The drawing under review shows one solid part. Ordinate dimensions are in mm from its lowest x, y, z. Coordinates: 2 decimals unless noted, no trailing zeros. Order: outer loops, then holes, each group sorted by start corner. A loop starts at its lowest first (then second) coordinate and runs counter-clockwise, first axis right, second up.
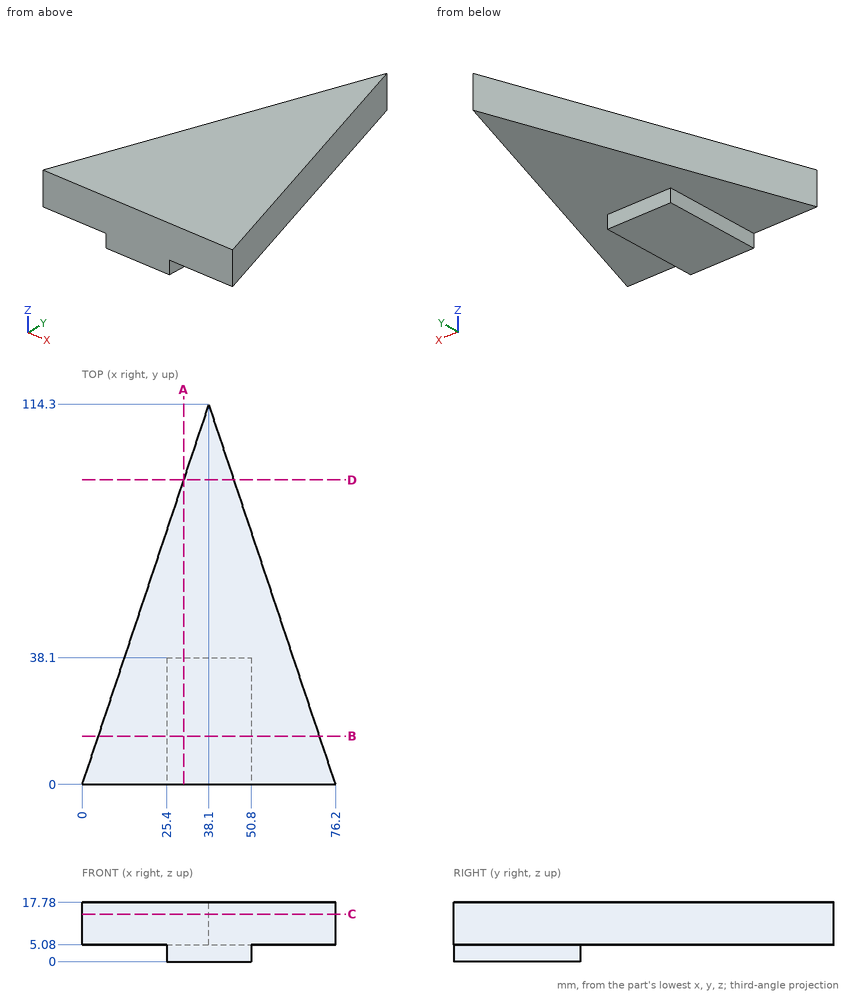
(1) Wall thickness on probe 1 along Y at (x, z) = (32, 3.75); probe 2 along Z at (x, y) = (55.5, 61.5); probe 3 along X at (y, z) = (34.5, 4.5): over which ranges is each line inside the solid? List them lowest first.
A:
probe 1: y = 0 to 38.1
probe 2: z = 5.08 to 17.78
probe 3: x = 25.4 to 50.8
(2) For pin 1 Ø6 at (y, z) = (17, 12) entering from -X; pin 2 Ø2 at (y, z) = (84.5, 12) entering from -X; pin 3 Ø5 at (y, z) = (82.5, 14.5) entering from +X, all flat-tipped, find the tip position at first contact; note any pin that passes through.
A:
pin 1: stops at x = 4.67
pin 2: stops at x = 27.83
pin 3: stops at x = 49.53
(3) We need section A-A, the plane x = 30.5. Write out the cut boundary in (y, z).
A:
outline: (0, 0) - (38.1, 0) - (38.1, 5.08) - (91.5, 5.08) - (91.5, 17.78) - (0, 17.78) - close
(4) We need section C-C, the plane z = 14.25. Write out the cut boundary in (x, y).
A:
outline: (0, 0) - (76.2, 0) - (38.1, 114.3) - close
(5) We need section B-B, the plane y = 14.5. Write out the cut boundary in (x, z).
A:
outline: (4.83, 5.08) - (25.4, 5.08) - (25.4, 0) - (50.8, 0) - (50.8, 5.08) - (71.37, 5.08) - (71.37, 17.78) - (4.83, 17.78) - close
(6) We need section D-D, the plane y = 91.5. Write out the cut boundary in (x, z), and give its area (3 significant figures).
A:
outline: (30.5, 5.08) - (45.7, 5.08) - (45.7, 17.78) - (30.5, 17.78) - close
area: 193 mm2
